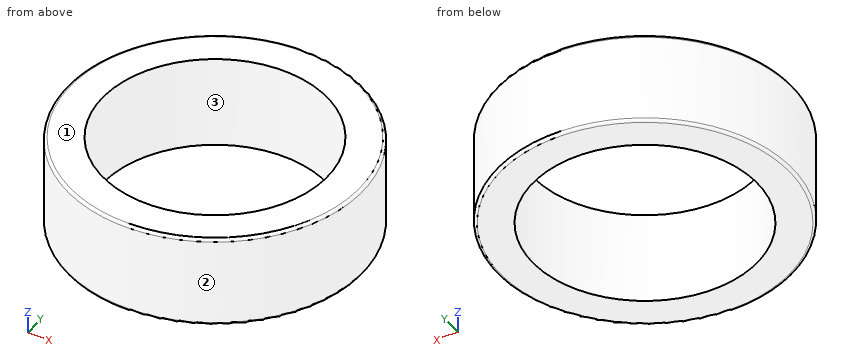
from build123d import *

# Parameters (mm, degrees)
CYLINDER002_R     = 6.1
CYLINDER002_DEPTH = 5
CYLINDER_R        = 8
CYLINDER_DEPTH    = 5
FILLET001_R       = 0.15


with BuildPart() as cilindro:
    # Cylinder002 → Cylinder002 (new body)
    with BuildSketch(Plane.XY):
        Circle(CYLINDER002_R)
    extrude(amount=CYLINDER002_DEPTH)


with BuildPart() as fillet001:
    # Cylinder → Cylinder (new body)
    with BuildSketch(Plane.XY):
        Circle(CYLINDER_R)
    extrude(amount=CYLINDER_DEPTH)

    # Cut: cut Cilindro
    add(cilindro.part, mode=Mode.SUBTRACT)

    # Fillet001
    fillet001_edges = [fillet001.edges().sort_by_distance(p)[0] for p in [
        (-8, 0, 0),
        (-8, 0, 5),
    ]]
    fillet(fillet001_edges, radius=FILLET001_R)


solid = fillet001.part
Input: part model. Units: mm. Frame: model coordinates. Face numbers are marked on the shaded views. Give positions to 0.01 mm unless a question says otherwise; leave off trailing zeros. Write each loop counter-clockwise with the first axis right and the second up, starting at its lowest first coordinate (ties: lowest second). Pieces come first, ordered by that corner, then holes. Notation, with made-up numbers: M 39,-19.5 L 68,-19.5 A18 cw 68,0.5 Z; hole C 83,-32.5 d11. An arc over 180 degrees is marked long. Write item = value, one per line. Start each with the question number.
1) Cut plane A-A on x = 0. Return the cut outline in (y, z), then the cut area to 3 significant figures.
2) Cut plane C-C on z = 1.5. Return the cut outline in (x, y), then the cut area to 3 significant figures.
3) Material intervals for line 1 along Y through (x, z) = (-0.25, 1.3); line 2 along Y through (x, z) = (-5, 1.25) (3 decimals); line 3 along X through (y, z) = (4.5, 1.2), sorted ascending. Write a range as [from, to].
4) Draft query along X for the marked faces 1, 2 and 3. Return one class per face: +X half, -X half, draft (parallel to the pull), parting line (faces both ways), or undercut.
Solved:
q1.outline = M -8,0.15 A0.15 ccw -7.85,0 L -6.1,0 L -6.1,5 L -7.85,5 A0.15 ccw -8,4.85 Z; M 6.1,0 L 7.85,0 A0.15 ccw 8,0.15 L 8,4.85 A0.15 ccw 7.85,5 L 6.1,5 Z
q1.area = 19.0 mm2
q2.outline = C 0,0 d16; hole C 0,0 d12.2
q2.area = 84.2 mm2
q3.line_1 = [-8, -6.09], [6.09, 8]
q3.line_2 = [-6.245, -3.494], [3.494, 6.245]
q3.line_3 = [-6.61, -4.12], [4.12, 6.61]
q4.face_1 = draft
q4.face_2 = parting line
q4.face_3 = undercut
